CAD build for the part. Positions are in the model's coordinates, mm. A direction names the side the tool comes from. Coordinates: 2 decimals unless noted, no trailing zeros. Answer in a Markdown table with one row per item. Add a question column.
Q1. Drill centre lines: line 1 along Y through (x, z) = (-17.5, 3.75); line 2 along Y through (x, z) = (-12, 3.75); line 3 along Y through (x, z) = (-13.5, 3.5). Where is each one in solid material? Low to high. Write a range as from..to.
Q2. Two-plate mould, pull along Y, no slides. Class faces 3 (the flat face through (-1, -25.4, 3)), 4 (the flat face through (12.834, -9, 3)), 5 (the flat face through (-1, 0, 6.35)): +Y half, -Y half, draft (parallel to the pull), parting line (faces both ways), or undercut.
Q3. Band-saw the part on A-A (z = 2). State how many separate pieces and enclosed holes the cut face has, and give its area (3 significant figures).
Q4. 3-axis set-ups, long thin cutter, end or side, ignore diameter. For faces 1 (the flat face through (-1, 0, 0)), 2 (the flat face through (-20, 3.64, 3)): which of +Z, -Z, +X, -X, +Y, -Y reach the whole face in a straight line?
```python
from build123d import *

# Parameters (mm, degrees)
F0_W     = 76.2
F0_H     = 50.8
F1_DEPTH = 6.35


with BuildPart() as f1:
    # F0 (on Top) → F1 (new body)
    with BuildSketch(Plane.XY):
        Rectangle(F0_W, F0_H)
        with BuildLine():
            Line((1.2140801556, -12.7), (-0.1628037906, -12.7))
            Line((-0.1628037906, -12.7), (-0.5311649502, -10.9547548942))
            Line((-0.5311649502, -10.9547548942), (-0.6205729987, -10.9547548942))
            add(Edge.make_bspline(
                [(-0.6205729987, -10.9547548942), (-1.5361114148, -12.1063305583), (-2.446285348, -12.5158194202)],
                knots=[0, 0, 0, 1, 1, 1], degree=2))
            add(Edge.make_bspline(
                [(-2.446285348, -12.5158194202), (-3.3564592813, -12.9253082821), (-4.7226142616, -12.9253082821)],
                knots=[0, 0, 0, 1, 1, 1], degree=2))
            add(Edge.make_bspline(
                [(-4.7226142616, -12.9253082821), (-6.5429621281, -12.9253082821), (-7.5765191682, -11.9847356124)],
                knots=[0, 0, 0, 1, 1, 1], degree=2))
            add(Edge.make_bspline(
                [(-7.5765191682, -11.9847356124), (-8.6100762083, -11.0441629427), (-8.6100762083, -9.3132231247)],
                knots=[0, 0, 0, 1, 1, 1], degree=2))
            add(Edge.make_bspline(
                [(-8.6100762083, -9.3132231247), (-8.6100762083, -5.6045772749), (-2.676958113, -5.425761178)],
                knots=[0, 0, 0, 1, 1, 1], degree=2))
            Line((-2.676958113, -5.425761178), (-0.599115067, -5.3578110612))
            Line((-0.599115067, -5.3578110612), (-0.599115067, -4.5960544884))
            add(Edge.make_bspline(
                [(-0.599115067, -4.5960544884), (-0.599115067, -3.1547967473), (-1.2178187623, -2.4681429352)],
                knots=[0, 0, 0, 1, 1, 1], degree=2))
            add(Edge.make_bspline(
                [(-1.2178187623, -2.4681429352), (-1.8365224576, -1.7814891231), (-3.2026774379, -1.7814891231)],
                knots=[0, 0, 0, 1, 1, 1], degree=2))
            add(Edge.make_bspline(
                [(-3.2026774379, -1.7814891231), (-4.7333432274, -1.7814891231), (-6.664557074, -2.7184854709)],
                knots=[0, 0, 0, 1, 1, 1], degree=2))
            Line((-6.664557074, -2.7184854709), (-7.236768584, -1.2986856615))
            add(Edge.make_bspline(
                [(-7.236768584, -1.2986856615), (-6.3319591337, -0.808729556), (-5.2536980694, -0.5297764448)],
                knots=[0, 0, 0, 1, 1, 1], degree=2))
            add(Edge.make_bspline(
                [(-5.2536980694, -0.5297764448), (-4.1754370051, -0.2508233337), (-3.0882351359, -0.2508233337)],
                knots=[0, 0, 0, 1, 1, 1], degree=2))
            add(Edge.make_bspline(
                [(-3.0882351359, -0.2508233337), (-0.8995261098, -0.2508233337), (0.1572770229, -1.2217947398)],
                knots=[0, 0, 0, 1, 1, 1], degree=2))
            add(Edge.make_bspline(
                [(0.1572770229, -1.2217947398), (1.2140801556, -2.192766146), (1.2140801556, -4.3385593088)],
                knots=[0, 0, 0, 1, 1, 1], degree=2))
            Line((1.2140801556, -4.3385593088), (1.2140801556, -12.7))
        make_face(mode=Mode.SUBTRACT)
        with BuildLine():
            Line((-22.246591758, -12.7), (-22.246591758, 3.6402149349))
            Line((-22.246591758, 3.6402149349), (-17.629560136, 3.6402149349))
            add(Edge.make_bspline(
                [(-17.629560136, 3.6402149349), (-14.3786834943, 3.6402149349), (-12.9249086265, 2.6674553678)],
                knots=[0, 0, 0, 1, 1, 1], degree=2))
            add(Edge.make_bspline(
                [(-12.9249086265, 2.6674553678), (-11.4711337587, 1.6946958006), (-11.4711337587, -0.404605177)],
                knots=[0, 0, 0, 1, 1, 1], degree=2))
            add(Edge.make_bspline(
                [(-11.4711337587, -0.404605177), (-11.4711337587, -1.8601682058), (-12.2811706777, -2.8043171974)],
                knots=[0, 0, 0, 1, 1, 1], degree=2))
            add(Edge.make_bspline(
                [(-12.2811706777, -2.8043171974), (-13.0912075966, -3.7484661891), (-14.6469076397, -4.0274193002)],
                knots=[0, 0, 0, 1, 1, 1], degree=2))
            Line((-14.6469076397, -4.0274193002), (-14.6469076397, -4.1382852803))
            add(Edge.make_bspline(
                [(-14.6469076397, -4.1382852803), (-10.9239565022, -4.7748705853), (-10.9239565022, -8.0507814805)],
                knots=[0, 0, 0, 1, 1, 1], degree=2))
            add(Edge.make_bspline(
                [(-10.9239565022, -8.0507814805), (-10.9239565022, -10.2394905066), (-12.4045537845, -11.4697452533)],
                knots=[0, 0, 0, 1, 1, 1], degree=2))
            add(Edge.make_bspline(
                [(-12.4045537845, -11.4697452533), (-13.8851510669, -12.7), (-16.5459345888, -12.7)],
                knots=[0, 0, 0, 1, 1, 1], degree=2))
            Line((-16.5459345888, -12.7), (-22.246591758, -12.7))
        make_face(mode=Mode.SUBTRACT)
        with BuildLine():
            Line((22.5003483308, -12.7), (20.6478135669, -12.7))
            Line((20.6478135669, -12.7), (20.6478135669, -4.731954722))
            add(Edge.make_bspline(
                [(20.6478135669, -4.731954722), (20.6478135669, -3.2656627274), (20.0219572278, -2.5343048911)],
                knots=[0, 0, 0, 1, 1, 1], degree=2))
            add(Edge.make_bspline(
                [(20.0219572278, -2.5343048911), (19.3961008886, -1.8029470548), (18.0764380935, -1.8029470548)],
                knots=[0, 0, 0, 1, 1, 1], degree=2))
            add(Edge.make_bspline(
                [(18.0764380935, -1.8029470548), (16.3454982755, -1.8029470548), (15.5175797468, -2.7971645535)],
                knots=[0, 0, 0, 1, 1, 1], degree=2))
            add(Edge.make_bspline(
                [(15.5175797468, -2.7971645535), (14.6896612181, -3.7913820523), (14.6896612181, -5.8584961325)],
                knots=[0, 0, 0, 1, 1, 1], degree=2))
            Line((14.6896612181, -5.8584961325), (14.6896612181, -12.7))
            Line((14.6896612181, -12.7), (12.8335501323, -12.7))
            Line((12.8335501323, -12.7), (12.8335501323, -4.731954722))
            add(Edge.make_bspline(
                [(12.8335501323, -4.731954722), (12.8335501323, -3.2656627274), (12.2076937931, -2.5343048911)],
                knots=[0, 0, 0, 1, 1, 1], degree=2))
            add(Edge.make_bspline(
                [(12.2076937931, -2.5343048911), (11.581837454, -1.8029470548), (10.251445693, -1.8029470548)],
                knots=[0, 0, 0, 1, 1, 1], degree=2))
            add(Edge.make_bspline(
                [(10.251445693, -1.8029470548), (8.5097769092, -1.8029470548), (7.6997399902, -2.8472330607)],
                knots=[0, 0, 0, 1, 1, 1], degree=2))
            add(Edge.make_bspline(
                [(7.6997399902, -2.8472330607), (6.8897030713, -3.8915190666), (6.8897030713, -6.2733494773)],
                knots=[0, 0, 0, 1, 1, 1], degree=2))
            Line((6.8897030713, -6.2733494773), (6.8897030713, -12.7))
            Line((6.8897030713, -12.7), (5.0335919854, -12.7))
            Line((5.0335919854, -12.7), (5.0335919854, -0.4510973622))
            Line((5.0335919854, -0.4510973622), (6.5427998433, -0.4510973622))
            Line((6.5427998433, -0.4510973622), (6.8432108861, -2.1283923511))
            Line((6.8432108861, -2.1283923511), (6.9326189345, -2.1283923511))
            add(Edge.make_bspline(
                [(6.9326189345, -2.1283923511), (7.4583382594, -1.2343118666), (8.4150043778, -0.7300504733)],
                knots=[0, 0, 0, 1, 1, 1], degree=2))
            add(Edge.make_bspline(
                [(8.4150043778, -0.7300504733), (9.3716704963, -0.2257890801), (10.5554330578, -0.2257890801)],
                knots=[0, 0, 0, 1, 1, 1], degree=2))
            add(Edge.make_bspline(
                [(10.5554330578, -0.2257890801), (13.427219574, -0.2257890801), (14.3105710927, -2.307208448)],
                knots=[0, 0, 0, 1, 1, 1], degree=2))
            Line((14.3105710927, -2.307208448), (14.3999791412, -2.307208448))
            add(Edge.make_bspline(
                [(14.3999791412, -2.307208448), (14.9471563977, -1.3451778467), (15.9860779207, -0.7854834634)],
                knots=[0, 0, 0, 1, 1, 1], degree=2))
            add(Edge.make_bspline(
                [(15.9860779207, -0.7854834634), (17.0249994437, -0.2257890801), (18.3553912046, -0.2257890801)],
                knots=[0, 0, 0, 1, 1, 1], degree=2))
            add(Edge.make_bspline(
                [(18.3553912046, -0.2257890801), (20.4332342506, -0.2257890801), (21.4667912907, -1.2933211786)],
                knots=[0, 0, 0, 1, 1, 1], degree=2))
            add(Edge.make_bspline(
                [(21.4667912907, -1.2933211786), (22.5003483308, -2.3608532771), (22.5003483308, -4.7104967904)],
                knots=[0, 0, 0, 1, 1, 1], degree=2))
            Line((22.5003483308, -4.7104967904), (22.5003483308, -12.7))
        make_face(mode=Mode.SUBTRACT)
    extrude(amount=F1_DEPTH)


solid = f1.part
```
Checked values:
| question | item | result |
|---|---|---|
| 1 | line 1 | y = -25.4..-12.7, 3.64..25.4 |
| 1 | line 2 | y = -25.4..-11.09, -5.29..-2.42, 1.72..25.4 |
| 1 | line 3 | y = -25.4..-12.14, -4.43..-3.69, 2.98..25.4 |
| 2 | face 3 | -Y half |
| 2 | face 4 | undercut |
| 2 | face 5 | draft |
| 3 | separate pieces | 1 |
| 3 | enclosed holes | 3 |
| 3 | area | 3,540 mm² |
| 4 | face 1 | -Z, +X, -X, +Y, -Y |
| 4 | face 2 | +Z, -Z |
